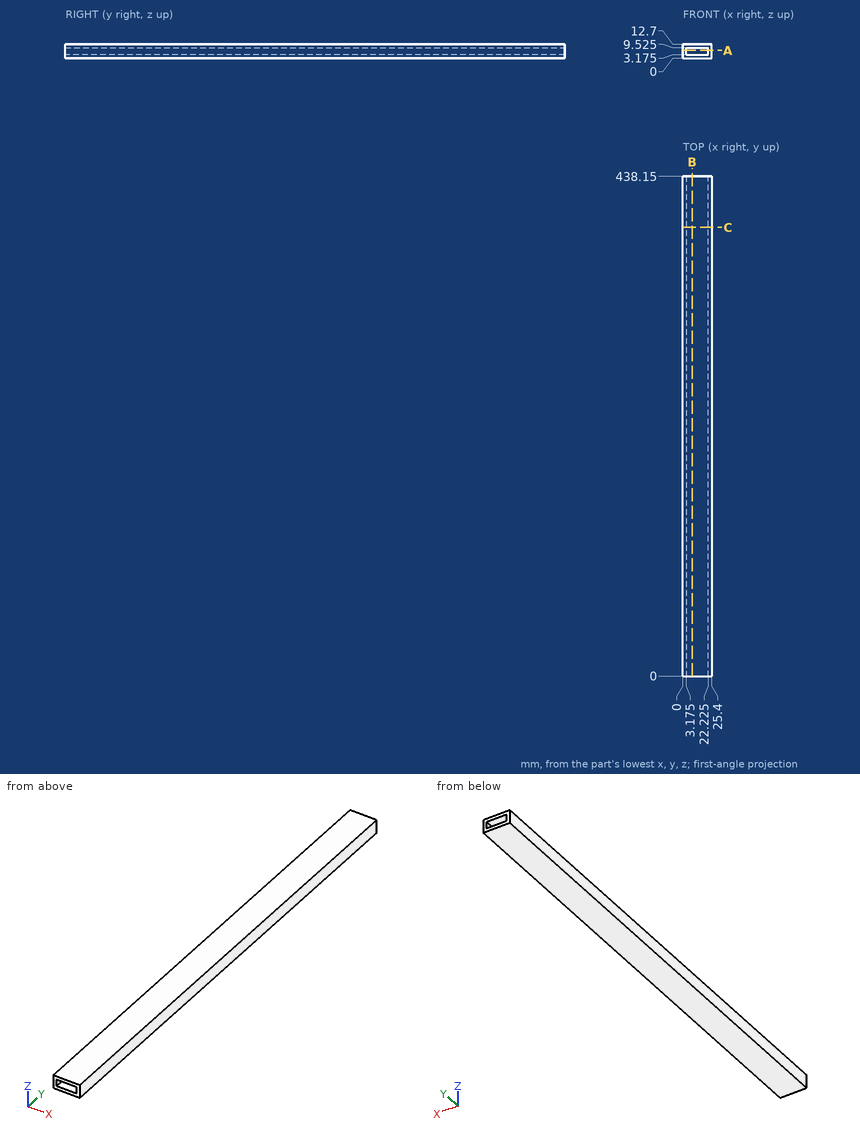
Design review of the part shown in the three views and the two pictorial views. Dimensions are in mm from the part's minimum x, y and z. Round coordinates to 2 decimals unless told otherwise and drop trailing zeros. Loops run counter-clockwise (first coordinate to the right, second up) from the corner with the lowest first, then second, coordinate; pieces in that order, holes last. Notation, with made-up numbers: (-7.75, -6.5) -> (23.25, -6.5) arc R27 ccw to (23.25, 21.5) -> close; hole circle Ø9 at (89, -37). An arc over 180 degrees is marked (long way). Use one line per item in the form item = value. Start each with the question number.
Q1. Wall thickness on line 1 along X through (y, z) = (348, 4) (3 decimals); line 2 along Z through (x, y) = (12.75, 195) (3 decimals): over which ranges is each line inside the solid? List them lowest first. Write a range as [from, to].
Q2. We need section B-B on x = 8.25. Give the boundary of the cut face in (y, z) (3 decimals), then the cut area to 3 significant figures.
Q3. We need section C-C on y = 393.5. Give the boundary of the cut face in (x, z) (3 decimals).
Q4. For pin 1 Ø3 at (x, z) = (8.5, 7.5) entering from -Y, flat-tipped, find the tip position at first contact; note if it passes through.
Q5. We need section A-A on z = 7. Give the boundary of the cut face in (x, y) (3 decimals).
Calculated:
q1.line_1 = [0, 3.175], [22.225, 25.4]
q1.line_2 = [0, 3.175], [9.525, 12.7]
q2.outline = (0, 0) -> (438.15, 0) -> (438.15, 3.175) -> (0, 3.175) -> close; (0, 9.525) -> (438.15, 9.525) -> (438.15, 12.7) -> (0, 12.7) -> close
q2.area = 2,780 mm²
q3.outline = (0, 0) -> (25.4, 0) -> (25.4, 12.7) -> (0, 12.7) -> close; hole (3.175, 3.175) -> (22.225, 3.175) -> (22.225, 9.525) -> (3.175, 9.525) -> close
q4.pin_1 = through
q5.outline = (0, 0) -> (3.175, 0) -> (3.175, 438.15) -> (0, 438.15) -> close; (22.225, 0) -> (25.4, 0) -> (25.4, 438.15) -> (22.225, 438.15) -> close
